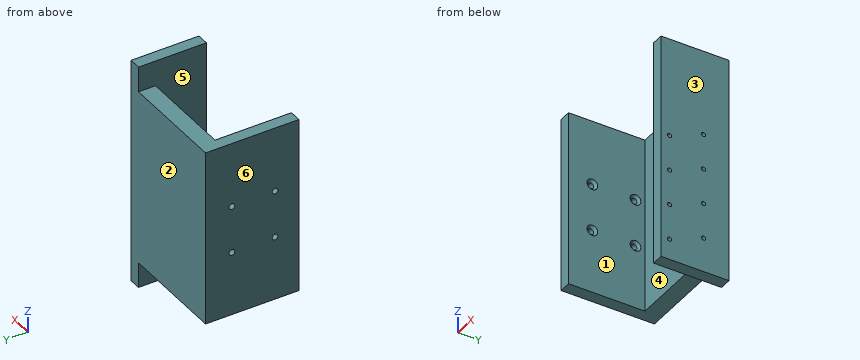
from build123d import *

# Parameters (mm, degrees)
SKETCH1_W                                           = 70
SKETCH1_H                                           = 55
BOSS_EXTRUDE1_DEPTH                                 = 134
CUT_EXTRUDE1_DEPTH                                  = 161.875728437
CUT_EXTRUDE1_DEPTH_BACK                             = 161.875728437
SKETCH4_R                                           = 1.25
CUT_EXTRUDE4_DEPTH                                  = 7
SKETCH5_W                                           = 14.985710671
SKETCH5_H                                           = 55
CUT_EXTRUDE5_DEPTH                                  = 63
CSK_FOR_M3_COUNTERSUNK_FLAT_HEAD_SCREW1_D           = 3.4
CSK_FOR_M3_COUNTERSUNK_FLAT_HEAD_SCREW1_DEPTH       = 10
CSK_FOR_M3_COUNTERSUNK_FLAT_HEAD_SCREW1_CSINK_D     = 6.3
CSK_FOR_M3_COUNTERSUNK_FLAT_HEAD_SCREW1_CSINK_ANGLE = 90
CSK_FOR_M3_COUNTERSUNK_FLAT_HEAD_SCREW1_TIP         = 1.021463052


with BuildPart() as part:
    # Sketch1 → Boss-Extrude1 (new body)
    with BuildSketch(Plane.XY):
        with Locations((35, 27.5)):
            Rectangle(SKETCH1_W, SKETCH1_H)
    extrude(amount=BOSS_EXTRUDE1_DEPTH)

    # Sketch2 → Cut-Extrude1 (cut, two sides: drawn at the far end of the back side and taken through both)
    with BuildSketch(Plane.XY.offset(134).offset(-CUT_EXTRUDE1_DEPTH_BACK)):
        Polygon((7, 0), (7, 45), (63, 45), (63, 15), (70, 15), (70, 0), (60, 0), align=None)
    extrude(amount=CUT_EXTRUDE1_DEPTH + CUT_EXTRUDE1_DEPTH_BACK, mode=Mode.SUBTRACT)

    # Sketch4 → Cut-Extrude4 (cut)
    with BuildSketch(Plane(origin=(70, 0, 0), x_dir=(0, 0, -1), z_dir=(1, 0, 0))):
        with Locations(Location((-83.331764561, 40, 0), (0, 0, 90))):
            Circle(SKETCH4_R)
        with Locations(Location((-75.331764561, 20, 0), (0, 0, 90))):
            Circle(SKETCH4_R)
        with Locations(Location((-62.331764561, 40, 0), (0, 0, 90))):
            Circle(SKETCH4_R)
        with Locations(Location((-54.331764561, 20, 0), (0, 0, 90))):
            Circle(SKETCH4_R)
        with Locations(Location((-41.331764561, 40, 0), (0, 0, 90))):
            Circle(SKETCH4_R)
        with Locations(Location((-33.331764561, 20, 0), (0, 0, 90))):
            Circle(SKETCH4_R)
        with Locations(Location((-20.331764561, 40, 0), (0, 0, 90))):
            Circle(SKETCH4_R)
        with Locations(Location((-12.331764561, 20, 0), (0, 0, 90))):
            Circle(SKETCH4_R)
    extrude(amount=-CUT_EXTRUDE4_DEPTH, mode=Mode.SUBTRACT)

    # Sketch5 → Cut-Extrude5 (cut)
    with BuildSketch(Plane.ZY):
        with Locations((7.492855336, 27.5)):
            Rectangle(SKETCH5_W, SKETCH5_H)
        with Locations((126.507144665, 27.5)):
            Rectangle(SKETCH5_W, SKETCH5_H)
    extrude(amount=-CUT_EXTRUDE5_DEPTH, mode=Mode.SUBTRACT)

    # CSK for M3 Countersunk Flat Head Screw1
    with Locations(Plane(origin=(7, 0, 0), x_dir=(0, 0, 1), z_dir=(1, 0, 0))):
        with Locations((52.691317064, -39.454373601), (52.691317064, -14.054373601), (80.631317064, -14.054373601), (80.631317064, -39.454373601)):
            CounterSinkHole(CSK_FOR_M3_COUNTERSUNK_FLAT_HEAD_SCREW1_D / 2, CSK_FOR_M3_COUNTERSUNK_FLAT_HEAD_SCREW1_CSINK_D / 2, depth=CSK_FOR_M3_COUNTERSUNK_FLAT_HEAD_SCREW1_DEPTH, counter_sink_angle=CSK_FOR_M3_COUNTERSUNK_FLAT_HEAD_SCREW1_CSINK_ANGLE)
            with Locations((0, 0, -(CSK_FOR_M3_COUNTERSUNK_FLAT_HEAD_SCREW1_DEPTH + CSK_FOR_M3_COUNTERSUNK_FLAT_HEAD_SCREW1_TIP / 2))):  # 118° drill point
                Cone(0, CSK_FOR_M3_COUNTERSUNK_FLAT_HEAD_SCREW1_D / 2, CSK_FOR_M3_COUNTERSUNK_FLAT_HEAD_SCREW1_TIP, mode=Mode.SUBTRACT)


solid = part.part
The listing builds one solid part. Answer for the finished solid, in the listing's coordinates (mm). Face numbers are marked on the shaded views. A direction names the side the tool comes from. Round coordinates to 2 decimals unless told otherwise and drop trailing zeros. Write each loop counter-clockwise with the first axis right and the second up, starting at its lowest first coordinate (ties: lowest second). Pieces come first, ordered by that corner, then holes. Notation, with made-up numbers: M 20.5,-12 L 56.5,-12 A28 ccw 56.5,12 Z; hole C 77,-11 d8. An arc over 180 degrees is marked long. Write each question's results on one line, items separated by ' | '. Start each with the question number.
Item 1: Which of the six approach directions +Z, -Z, +X, -X, +Y, -Y give full straight-line access (tool end or side, diameter ignored) to the marked faces 1 and 2?
Item 2: Given pin 1 Ø4.5 at (y, z) = (39.45, 52.69) entering from -X; pin 2 Ø2.5 at (y, z) = (39.45, 80.63) entering from -X; pin 3 Ø2 at (y, z) = (40, 41.33) entering from +X; pin 4 Ø3.5 at (x, z) = (65.5, 73) entering from -Y, each flat-ended and moving along its own axis, determine where each tip first touches the part or whether it passes through.
Item 3: Find section C-C on y = 48. Write down the section's boundary in (x, z).
Item 4: Find section D-D on x = 52.5. Write down the section's boundary in (y, z), and give its area (3 significant figures).
Item 5: Find section A-A on y = 34.5. Write down the section's boundary in (x, z).
Item 6: Straight lines are drawn through the part: probe 1 along Z at (x, y) = (68, 40); probe 2 along Z at (x, y) = (65.25, 20); probe 3 along X at (y, z) = (30.5, 68.5). For each, find the intervals that lie inside material, in ascending order.
Item 7: Find section B-B on z = 106. Write down the section's boundary in (x, y).
Item 8: The mould has two halves that part along X. Classify the marked faces 3, 4, 5 and 6: +X half, -X half, draft (parallel to the pull), parting line (faces both ways), or undercut.
Answer block:
1) face 1: +Z, -Z, -Y | face 2: +Z, -Z, +X, -X, +Y
2) pin 1: stops at x = 0 | pin 2: stops at x = 63 | pin 3: stops at x = 7 | pin 4: stops at y = 15
3) outline: M 0,14.99 L 63,14.99 L 63,0 L 70,0 L 70,134 L 63,134 L 63,119.01 L 0,119.01 Z
4) outline: M 45,14.99 L 55,14.99 L 55,119.01 L 45,119.01 Z | area: 1,040 mm²
5) outline: M 0,14.99 L 7,14.99 L 7,119.01 L 0,119.01 Z; M 63,0 L 70,0 L 70,134 L 63,134 Z
6) probe 1: z = 0 to 19.08, 21.58 to 40.08, 42.58 to 61.08, 63.58 to 82.08, 84.58 to 134 | probe 2: z = 0 to 11.08, 13.58 to 32.08, 34.58 to 53.08, 55.58 to 74.08, 76.58 to 134 | probe 3: x = 0 to 7, 63 to 70
7) outline: M 0,0 L 7,0 L 7,45 L 63,45 L 63,15 L 70,15 L 70,55 L 0,55 Z
8) face 3: +X half | face 4: undercut | face 5: undercut | face 6: -X half
